Design review of the part shown in the three views and the two pictorial views. Dimensions are in mm from the part's minimum x, y and z. A direction names the side the tool comes from. Give positions to 0.01 mm unless a question says otherwise; leave off trailing zeros. Order: outer loops, then holes, each group sorted by start corner. A loop starts at its lowest first (then second) coordinate and runs counter-clockwise, first axis right, second up.
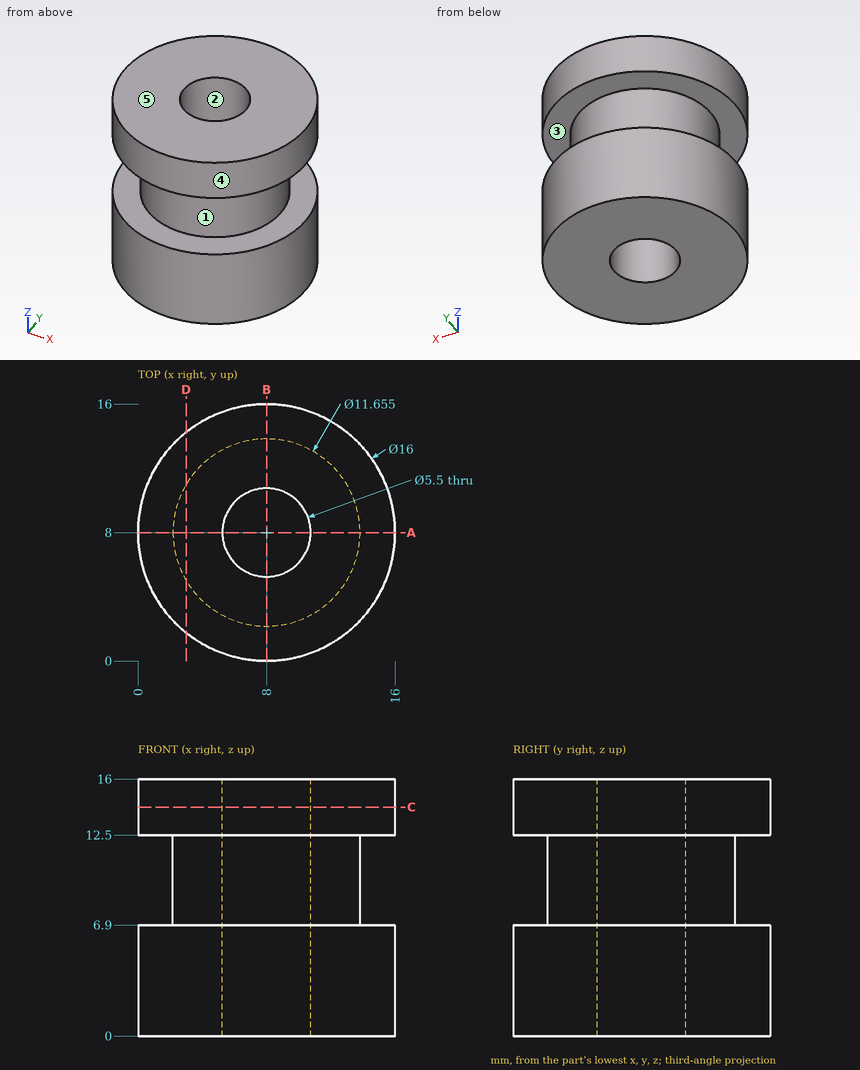
1) We need section D-D on x = 3. Give the boundary of the cut face in (y, z) (3 decimals), then the cut area to 3 significant figures.
Answer sheet:
outline: (1.755, 0) - (14.245, 0) - (14.245, 6.9) - (10.993, 6.9) - (10.993, 12.5) - (14.245, 12.5) - (14.245, 16) - (1.755, 16) - (1.755, 12.5) - (5.007, 12.5) - (5.007, 6.9) - (1.755, 6.9) - close
area: 163 mm2
2) Clearance check with flat-ended pins moving along their axes: pin 1 (3 mm diameter, centred on y = 10.5, z = 3, fed in from +X); pin 2 (1.5 mm diameter, centred on x = 12, z = 13, fed in from -Y); pin 3 (5 mm diameter, centred on x = 5, y = 7, fed in from -Z); pin 4 (5 mm diameter, centred on x = 3, z = 1.5, fed in from +Y). State where each tip first meets the part, or that it passes through.
Answer sheet:
pin 1: stops at x = 15.94
pin 2: stops at y = 0.69
pin 3: stops at z = 0
pin 4: stops at y = 15.6
3) We need section C-C on z = 14.25. Give the boundary of the cut face in (x, y).
Answer sheet:
outline: circle Ø16 at (8, 8); hole circle Ø5.5 at (8, 8)
4) Draft analysis for pull direction Z (two halves, no side actions). For the marked faces 3, 4 and 5, state which applies: +Z half, -Z half, draft (parallel to the pull), parting line (faces both ways), or undercut.
Answer sheet:
face 3: undercut
face 4: draft
face 5: +Z half
5) We need section A-A on y = 8. Give the boundary of the cut face in (x, z).
Answer sheet:
outline: (0, 0) - (5.25, 0) - (5.25, 16) - (0, 16) - (0, 12.5) - (2.17, 12.5) - (2.17, 6.9) - (0, 6.9) - close; (10.75, 0) - (16, 0) - (16, 6.9) - (13.83, 6.9) - (13.83, 12.5) - (16, 12.5) - (16, 16) - (10.75, 16) - close
6) Tool access review of the marked faces 1 and 2: name each direction out of +Z, -Z, +X, -X, +Y, -Y from which nothing blocks a thin tool from reaching the whole face with its end or side.
Answer sheet:
face 1: none
face 2: +Z, -Z
7) To check wall thickness, follow line 1 (Y direction, x = 8, z = 15.5); line 2 (Y direction, x = 8, z = 8.5). State the ranges of each line that lie inside material, in increasing order.
Answer sheet:
line 1: y = 0 to 5.25, 10.75 to 16
line 2: y = 2.17 to 5.25, 10.75 to 13.83
